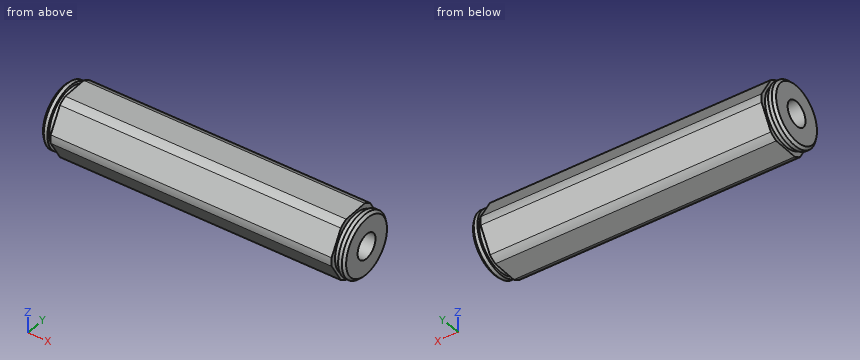
```python
from build123d import *

# Parameters (mm, degrees)
CUT_EXTRUDE1_START = 2.2606
SKETCH2_OUTSIDE_W  = 30.324
SKETCH2_OUTSIDE_H  = 30.324
CUT_EXTRUDE1_DEPTH = 57.2516
SKETCH5_R          = 2.5527
CUT_EXTRUDE2_DEPTH = 61.7728
CHAMFER1_SIZE      = 0.508


with BuildPart() as part:
    # Sketch4 → Revolve1 (revolve)
    with BuildSketch(Plane(origin=(0, 0, 0), x_dir=(1, 0, 0), z_dir=(0, 1, 0)), mode=Mode.PRIVATE) as revolve1_sk:
        Polygon((1.27, 6.35), (1.27, 5.842), (2.2606, 5.842), (2.2606, 7.62), (59.5122, 7.62), (59.5122, 5.842), (60.5028, 5.842), (60.5028, 6.35), (61.7728, 6.35), (61.7728, 0), (0, 0), (0, 6.35), align=None)
    revolve(revolve1_sk.sketch.rotate(Axis((0, 0, 0), (1, 0, 0)), 180), axis=Axis((0, 0, 0), (1, 0, 0)))

    # Sketch2 outside → Cut-Extrude1 (cut)
    with BuildSketch(Plane(origin=(0, 0, 0), x_dir=(0, 0, -1), z_dir=(1, 0, 0)).offset(CUT_EXTRUDE1_START)):
        Rectangle(SKETCH2_OUTSIDE_W, SKETCH2_OUTSIDE_H)
        with BuildLine():
            Line((5.456960506, 4.181770802), (0.893039494, 6.816751826))
            ThreePointArc((0.893039494, 6.816751826), (0, 6.875), (-0.893039494, 6.816751826))
            Line((-0.893039494, 6.816751826), (-5.456960506, 4.181770802))
            ThreePointArc((-5.456960506, 4.181770802), (-5.953924651, 3.4375), (-6.35, 2.634981025))
            Line((-6.35, 2.634981025), (-6.35, -2.634981025))
            ThreePointArc((-6.35, -2.634981025), (-5.953924651, -3.4375), (-5.456960506, -4.181770802))
            Line((-5.456960506, -4.181770802), (-0.893039494, -6.816751826))
            ThreePointArc((-0.893039494, -6.816751826), (0, -6.875), (0.893039494, -6.816751826))
            Line((0.893039494, -6.816751826), (5.456960506, -4.181770802))
            ThreePointArc((5.456960506, -4.181770802), (5.953924651, -3.4375), (6.35, -2.634981025))
            Line((6.35, -2.634981025), (6.35, 2.634981025))
            ThreePointArc((6.35, 2.634981025), (5.953924651, 3.4375), (5.456960506, 4.181770802))
        make_face(mode=Mode.SUBTRACT)
    extrude(amount=CUT_EXTRUDE1_DEPTH, mode=Mode.SUBTRACT)

    # Sketch5 → Cut-Extrude2 (cut)
    with BuildSketch(Plane(origin=(61.7728, 0, 0), x_dir=(0, 0, -1), z_dir=(1, 0, 0))):
        Circle(SKETCH5_R)
    extrude(amount=-CUT_EXTRUDE2_DEPTH, mode=Mode.SUBTRACT)

    # Chamfer1
    chamfer1_edges = [part.edges().sort_by_distance(p)[0] for p in [
        (0, 0, -6.35),
        (61.7728, 0, -6.35),
    ]]
    chamfer(chamfer1_edges, length=CHAMFER1_SIZE)


solid = part.part
```
Geometry: final body of the model. Coordinates: model frame, mm. Coordinates: 2 decimals unless noted, no trailing zeros. Order: outer loops, then holes, each group sorted by start corner. A loop starts at its lowest first (then second) coordinate and runs counter-clockwise, first axis right, second up. Notation, with made-up numbers: (-29, -20) - (-1, -20) arc R16 ccw to (-1, 4) - close; hole circle Ø8 at (-4.75, -25). An arc over 180 degrees is marked (long way). Write each question's results on one line, items separated by ' | '.
1) Section B-B, the plane x = 11. Return loops of the section in (y, z) (3 decimals).
Results list:
outline: (-6.817, -0.893) - (-4.182, -5.457) arc R6.875 ccw to (-2.635, -6.35) - (2.635, -6.35) arc R6.875 ccw to (4.182, -5.457) - (6.817, -0.893) arc R6.875 ccw to (6.817, 0.893) - (4.182, 5.457) arc R6.875 ccw to (2.635, 6.35) - (-2.635, 6.35) arc R6.875 ccw to (-4.182, 5.457) - (-6.817, 0.893) arc R6.875 ccw to start; hole circle Ø5.105 at (0, 0)
2) Section A-A, the plane y = 0. Return loops of the section in (x, z).
Results list:
outline: (0, -5.84) - (0.51, -6.35) - (1.27, -6.35) - (1.27, -5.84) - (2.26, -5.84) - (2.26, -6.35) - (59.51, -6.35) - (59.51, -5.84) - (60.5, -5.84) - (60.5, -6.35) - (61.26, -6.35) - (61.77, -5.84) - (61.77, -2.55) - (0, -2.55) - close; (0, 2.55) - (61.77, 2.55) - (61.77, 5.84) - (61.26, 6.35) - (60.5, 6.35) - (60.5, 5.84) - (59.51, 5.84) - (59.51, 6.35) - (2.26, 6.35) - (2.26, 5.84) - (1.27, 5.84) - (1.27, 6.35) - (0.51, 6.35) - (0, 5.84) - close
3) Section C-C, the plane z = 0. Return loops of the section in (x, y) (3 decimals).
Results list:
outline: (0, -5.842) - (0.508, -6.35) - (1.27, -6.35) - (1.27, -5.842) - (2.261, -5.842) - (2.261, -6.875) - (59.512, -6.875) - (59.512, -5.842) - (60.503, -5.842) - (60.503, -6.35) - (61.265, -6.35) - (61.773, -5.842) - (61.773, -2.553) - (0, -2.553) - close; (0, 2.553) - (61.773, 2.553) - (61.773, 5.842) - (61.265, 6.35) - (60.503, 6.35) - (60.503, 5.842) - (59.512, 5.842) - (59.512, 6.875) - (2.261, 6.875) - (2.261, 5.842) - (1.27, 5.842) - (1.27, 6.35) - (0.508, 6.35) - (0, 5.842) - close
4) Pin query (flat end, axial travel): pin 1 (3 mm diameter, centred on y = -1, z = 0, fed in from +X); pin 2 (2 mm diameter, centred on y = -5, z = 5, fed in from +X); pin 3 (1 mm diameter, centred on x = 22.5, z = 1, fed in from +Y); pin 4 (5 mm diameter, centred on x = 7, z = -3, fed in from -Y). Return the tip coordinate at first contact, or that it passes through.
Results list:
pin 1: through | pin 2: x = 61.54 | pin 3: y = 6.86 | pin 4: y = -6.86
5) Line query: line 1 (Y direction, x = 30, z = 0) (3 decimals); line 2 (X direction, y = -3.5, z = 5); line 3 (X direction, y = 5.25, z = 3.5). Output: solid intervals per line, ascending. Write a range as from..to.
Results list:
line 1: -6.875..-2.553, 2.553..6.875 | line 2: 0.26..1.27, 2.26..59.51, 60.5..61.51 | line 3: 0.47..1.27, 2.26..59.51, 60.5..61.31
